Check sheet for the modelled part. Datum: model origin and axes. Units: mm. A direction names the side the tool comes from. Round coordinates to 2 decimals unless told otherwise and drop trailing zeros. Write each loop counter-clockwise with the first axis right and the second up, starting at its lowest first coordinate (ties: lowest second). Pieces come first, ordered by that corner, then holes. Notation, with made-up numbers: (-36, 67) - (-16, 67) arc R20 cw to (-16, 87) - close; hole circle Ø2 at (63, 53.25). An arc over 180 degrees is marked (long way). Use one line per item in the form item = value. Start each with the question number.
1) Section check A-A (x = 50). Record the boundary of the cut face in (y, z), then the cut area to 3 significant figures.
2) Scan lines: probe 1 along X at (y, z) = (5.75, -10); probe 2 along X at (y, z) = (5.25, 20); probe 3 along Z at (x, y) = (-50.5, 3.25). Record each from-to range of solid material in increasing order.
3) Set-up check for faces 4 (the face through (-14.1, 2.47, 3.79)), 5 (the face through (0, 0, 18)), 6 (the face through (22.17, 3.45, -19.76)): record each of +Z, -Z, +X, -X, +Y, -Y from which the full face is reachable in a straight line by a thin tool's end or side.
4) Section check D-D (y = 3.75). Record the boundary of the cut face in (x, z).
5) Section check B-B (x = -20). Record the boundary of the cut face in (y, z).
6) Draft check along Z on faces 1 (the face through (0, 2, -10)), 2 (the face through (25, 7, -12)), 3 (the face through (0, 2, -5)). Enter one of: +Z half, -Z half, draft (parallel to the pull), parting line (faces both ways), or undercut.
7) Section check C-C (z = -7.5). Record the boundary of the cut face in (x, y), then the cut area to 3 significant figures.
8) Gauge pin test, flat ends, axial feed: P1, Ø4, axis at x = 2.5, y = 5, coming from the +Z side; P2, Ø2.5, axis at x = 1, y = 2.5, coming from the -Z side; P3, Ø2, axis at x = -42.5, y = 3, coming from the -Z side. Record the tip position at first contact, or that the pin passes through.
from build123d import *

# Parameters (mm, degrees)
SKETCH1_R               = 5
BOSS_EXTRUDE1_DEPTH     = 5
SKETCH1_3_R             = 10
SKETCH1_3_R_2           = 5
BOSS_EXTRUDE2_DEPTH     = 7
CUT_EXTRUDE1_DEPTH      = 68.268120235
CUT_EXTRUDE1_DEPTH_BACK = 68.268120235


with BuildPart() as part:
    # Sketch1 → Boss-Extrude1 (new body)
    with BuildSketch(Plane(origin=(0, 0, 0), x_dir=(1, 0, 0), z_dir=(0, 1, 0))):
        with BuildLine():
            ThreePointArc((-10, 10), (-23.826834324, 19.238795325), (-27.071067812, 2.928932188))
            Line((-27.071067812, 2.928932188), (-42.928932188, -12.928932188))
            ThreePointArc((-42.928932188, -12.928932188), (-59.238795325, -23.826834324), (-40, -20))
            Line((-40, -20), (40, -20))
            ThreePointArc((40, -20), (59.238795325, -23.826834324), (42.928932188, -12.928932188))
            Line((42.928932188, -12.928932188), (27.071067812, 2.928932188))
            ThreePointArc((27.071067812, 2.928932188), (23.826834324, 19.238795325), (10, 10))
            Line((10, 10), (-10, 10))
        make_face()
        with Locations(Location((-20, 10, 0), (0, 0, 270))):
            Circle(SKETCH1_R, mode=Mode.SUBTRACT)
        with Locations(Location((50, -20, 0), (0, 0, 270))):
            Circle(SKETCH1_R, mode=Mode.SUBTRACT)
        with Locations(Location((-50, -20, 0), (0, 0, 270))):
            Circle(SKETCH1_R, mode=Mode.SUBTRACT)
        with Locations(Location((20, 10, 0), (0, 0, 270))):
            Circle(SKETCH1_R, mode=Mode.SUBTRACT)
    extrude(amount=BOSS_EXTRUDE1_DEPTH)

    # Sketch1_3 → Boss-Extrude2 (add)
    # profile 1 of 4: a face of its own
    with BuildSketch(Plane(origin=(0, 0, 0), x_dir=(1, 0, 0), z_dir=(0, 1, 0))):
        with Locations(Location((-50, -20, 0), (0, 0, 45))):
            Circle(SKETCH1_3_R)
        with Locations(Location((-50, -20, 0), (0, 0, 270))):
            Circle(SKETCH1_3_R_2, mode=Mode.SUBTRACT)
    # profile 2 of 4: a face of its own
    with BuildSketch(Plane(origin=(0, 0, 0), x_dir=(1, 0, 0), z_dir=(0, 1, 0))):
        with Locations((-20, 10)):
            Circle(SKETCH1_3_R)
        with Locations(Location((-20, 10, 0), (0, 0, 270))):
            Circle(SKETCH1_3_R_2, mode=Mode.SUBTRACT)
    # profile 3 of 4: a face of its own
    with BuildSketch(Plane(origin=(0, 0, 0), x_dir=(1, 0, 0), z_dir=(0, 1, 0))):
        with Locations(Location((20, 10, 0), (0, 0, 180))):
            Circle(SKETCH1_3_R)
        with Locations(Location((20, 10, 0), (0, 0, 270))):
            Circle(SKETCH1_3_R_2, mode=Mode.SUBTRACT)
    # profile 4 of 4: a face of its own
    with BuildSketch(Plane(origin=(0, 0, 0), x_dir=(1, 0, 0), z_dir=(0, 1, 0))):
        with Locations(Location((50, -20, 0), (0, 0, 135))):
            Circle(SKETCH1_3_R)
        with Locations(Location((50, -20, 0), (0, 0, 270))):
            Circle(SKETCH1_3_R_2, mode=Mode.SUBTRACT)
    extrude(amount=BOSS_EXTRUDE2_DEPTH)

    # Sketch3 → Cut-Extrude1 (cut, two sides: drawn at the far end of the back side and taken through both)
    with BuildSketch(Plane(origin=(0, 5, 0), x_dir=(1, 0, 0), z_dir=(0, 1, 0)).offset(-CUT_EXTRUDE1_DEPTH_BACK)):
        with BuildLine():
            Line((-35.857864376, -15), (35.857864376, -15))
            ThreePointArc((35.857864376, -15), (36.141807012, -14.259748515), (36.464466094, -13.535533906))
            Line((36.464466094, -13.535533906), (26.464466094, -3.535533906))
            ThreePointArc((26.464466094, -3.535533906), (14.259748515, -3.858192988), (5.857864376, 5))
            Line((5.857864376, 5), (-5.857864376, 5))
            ThreePointArc((-5.857864376, 5), (-14.259748515, -3.858192988), (-26.464466094, -3.535533906))
            Line((-26.464466094, -3.535533906), (-36.464466094, -13.535533906))
            ThreePointArc((-36.464466094, -13.535533906), (-36.141807012, -14.259748515), (-35.857864376, -15))
        make_face()
    extrude(amount=CUT_EXTRUDE1_DEPTH + CUT_EXTRUDE1_DEPTH_BACK, mode=Mode.SUBTRACT)


solid = part.part
Results are:
q1.outline = (0, 10) - (7, 10) - (7, 15) - (0, 15) - close; (0, 25) - (7, 25) - (7, 30) - (0, 30) - close
q1.area = 70.0 mm²
q2.probe_1 = -30 to -25, -15 to -10, 10 to 15, 25 to 30
q2.probe_2 = -60 to -55, -45 to -40, 40 to 45, 55 to 60
q2.probe_3 = 10.01 to 15.03, 24.97 to 29.99
q3.face_4 = +Y, -Y
q3.face_5 = +Z, -Z, +X, -X, -Y
q3.face_6 = +Y
q4.outline = (-42.93, 12.93) - (-27.07, -2.93) arc R10 ccw (long way) to (-10, -10) - (10, -10) arc R10 ccw (long way) to (27.07, -2.93) - (42.93, 12.93) arc R10 ccw (long way) to (40, 20) - (-40, 20) arc R10 ccw (long way) to start; hole circle Ø10 at (-50, 20); hole (-36.46, 13.54) - (-26.46, 3.54) arc R15 cw to (-5.86, -5) - (5.86, -5) arc R15 cw to (26.46, 3.54) - (36.46, 13.54) arc R15 cw to (35.86, 15) - (-35.86, 15) arc R15 cw to start; hole circle Ø10 at (-20, -10); hole circle Ø10 at (20, -10); hole circle Ø10 at (50, 20)
q5.outline = (0, -20) - (7, -20) - (7, -15) - (0, -15) - close; (0, -5) - (7, -5) - (7, 0) - (5, 0) - (5, 5) - (0, 5) - close; (0, 15) - (5, 15) - (5, 20) - (0, 20) - close
q6.face_1 = -Z half
q6.face_2 = draft
q6.face_3 = undercut
q7.outline = (-29.68, 0) - (-24.33, 0) - (-24.33, 7) - (-29.68, 7) - close; (-15.67, 0) - (15.67, 0) - (15.67, 7) - (10.32, 7) - (10.32, 5) - (-10.32, 5) - (-10.32, 7) - (-15.67, 7) - close; (24.33, 0) - (29.68, 0) - (29.68, 7) - (24.33, 7) - close
q7.area = 253 mm²
q8.P1 = 20
q8.P2 = -10
q8.P3 = 11.5
